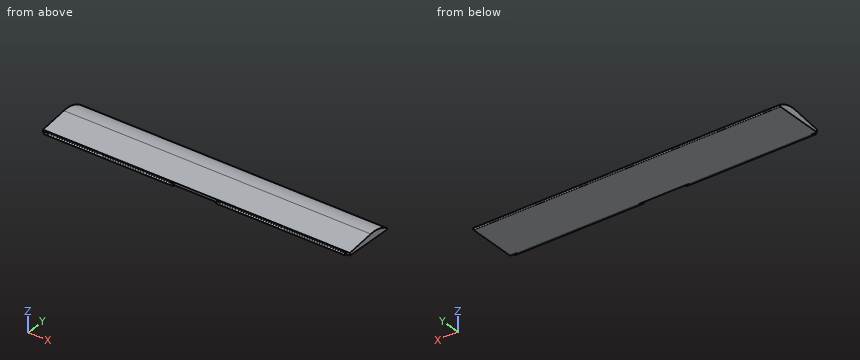
```python
from build123d import *

# Parameters (mm, degrees)
PAD021_DEPTH    = 250
SKETCH046_W     = 3.12
SKETCH046_H     = 200
PAD022_DEPTH    = 4.62
SKETCH047_R     = 1.56
PAD023_DEPTH    = 5
SKETCH048_R     = 1.56
PAD024_DEPTH    = 5
SKETCH049_R     = 1.56
PAD025_DEPTH    = 5
SKETCH050_R     = 1.56
PAD026_DEPTH    = 5
POCKET024_DEPTH = 480


with BuildPart() as part:
    # Sketch045 → Pad021 (new body, symmetric)
    with BuildSketch(Plane.YZ):
        with BuildLine():
            ThreePointArc((79.416029, -1.367224), (62.968794, 5.906774), (45, 6.645022))
            Line((0, 0), (45, 6.645022))
            Line((0, 0), (0, -4.12))
            Line((0, -4.12), (78.558353, -4.12))
            ThreePointArc((78.558353, -4.12), (80, -3.059171), (79.416029, -1.367224))
        make_face()
    extrude(amount=PAD021_DEPTH, both=True)

    # Sketch046 (on Face3 of Pad021) → Pad022 (join)
    with BuildSketch(Plane(origin=(0, 0, 0), x_dir=(0, 0, -1), z_dir=(0, -1, 0))):
        with Locations((2.06, 140)):
            Rectangle(SKETCH046_W, SKETCH046_H)
        with Locations((2.06, -140)):
            Rectangle(SKETCH046_W, SKETCH046_H)
    extrude(amount=PAD022_DEPTH)

    # Sketch047 (on Face11 of Pad022) → Pad023 (join)
    with BuildSketch(Plane.YZ.offset(240)):
        with Locations((-3.06, -2.06)):
            Circle(SKETCH047_R)
    extrude(amount=PAD023_DEPTH)

    # Sketch048 (on Face9 of Pad023) → Pad024 (join)
    with BuildSketch(Plane(origin=(40, 0, 0), x_dir=(0, 1, 0), z_dir=(-1, 0, 0))):
        with Locations((-3.06, 2.06)):
            Circle(SKETCH048_R)
    extrude(amount=PAD024_DEPTH)

    # Sketch049 (on Face15 of Pad024) → Pad025 (join)
    with BuildSketch(Plane.YZ.offset(-40)):
        with Locations((-3.06, -2.06)):
            Circle(SKETCH049_R)
    extrude(amount=PAD025_DEPTH)

    # Sketch050 (on Face13 of Pad025) → Pad026 (join)
    with BuildSketch(Plane(origin=(-240, 0, 0), x_dir=(0, 1, 0), z_dir=(-1, 0, 0))):
        with Locations((-3.06, 2.06)):
            Circle(SKETCH050_R)
    extrude(amount=PAD026_DEPTH)

    # Sketch052 (on Face13 of Pad026) → Pocket024 (cut)
    with BuildSketch(Plane(origin=(-240, 0, 0), x_dir=(0, 1, 0), z_dir=(-1, 0, 0))):
        with BuildLine():
            ThreePointArc((-3.06, 3.62), (-4.619996, 2.06), (-3.06, 0.5))
            Line((-4.62, 0.5), (-3.06, 0.5))
            Line((-4.62, 3.62), (-4.62, 0.5))
            Line((-4.62, 3.62), (-3.06, 3.62))
        make_face()
    extrude(amount=-POCKET024_DEPTH, mode=Mode.SUBTRACT)


solid = part.part
```
For this review, take the finished solid that the model builds, in its own axes (mm). Coordinates: 2 decimals unless noted, no trailing zeros. Order: outer loops, then holes, each group sorted by start corner. A loop starts at its lowest first (then second) coordinate and runs counter-clockwise, first axis right, second up. Notation, with made-up numbers: (15, -18) - (62, -18) arc R13 cw to (62, 5) - close; hole circle Ø8 at (-38, 13). An arc over 180 degrees is marked (long way). Answer as a JSON object with one key per item and string values. Group by question number.
1. We need section D-D on y = 16.5. State the section outline as (x, z) points, then the cut area to 3 significant figures.
2. For probe 1 along Y at (x, z) = (86, -2.5); probe 2 along Y at (x, z) = (-39, -2); probe 3 along Z at (x, y) = (57.5, 5), list the stretches that pass through material, from the lowest coordinate up.
3. Clearance check with flat-ended pins moving along their axes: P1, Ø2, axis at x = 187, z = -0.5, coming from the -Y side; P2, Ø3.5, axis at y = -2, z = -1.5, coming from the -X side; P3, Ø1, axis at x = 64, y = 60.5, coming from the +Z side. State where each tip first meets the part, or that it passes through.
4. We need section A-A on x = 197. State the section outline as (y, z) points, then the cut area to 3 significant figures.
5. We need section C-C on x = 25.5. State the section outline as (y, z) points, then the cut area to 3 significant figures.
6. We need section B-B on y = 36.5. State the section outline as (x, z) points, then the cut area to 3 significant figures.
Final values:
{
 "1": {"outline": "(-250, -4.12) - (250, -4.12) - (250, 2.44) - (-250, 2.44) - close", "area": "3,280 mm²"},
 "2": {"probe 1": "-4.56 to 80.06", "probe 2": "-4.62 to -1.5, 0 to 79.94", "probe 3": "-4.12 to 0.74"},
 "3": {"P1": "y = -4.52", "P2": "x = -245", "P3": "z = 6.5"},
 "4": {"outline": "(-3.06, -3.62) - (0, -3.62) - (0, -4.12) - (78.56, -4.12) arc R1.51 ccw to (79.42, -1.37) arc R48.2 ccw to (45, 6.65) - (0, 0) - (0, -0.5) - (-3.06, -0.5) arc R1.56 ccw to start", "area": "662 mm²"},
 "5": {"outline": "(0, -4.12) - (78.56, -4.12) arc R1.51 ccw to (79.42, -1.37) arc R48.2 ccw to (45, 6.65) - (0, 0) - close", "area": "648 mm²"},
 "6": {"outline": "(-250, -4.12) - (250, -4.12) - (250, 5.39) - (-250, 5.39) - close", "area": "4,750 mm²"}
}
